Read the model definition and answer for the solid it produces. Units are mm, in the model's axes. A direction names the side the tool comes from. Give positions to 0.01 mm unless a question says otherwise; leave off trailing zeros. Order: outer loops, then holes, each group sorted by start corner. A loop starts at its lowest first (then second) coordinate and runs counter-clockwise, first axis right, second up. Notation, with made-up numbers: (17, -6.75) - (59, -6.75) arc R27 ccw to (59, 14.25) - close; hole circle Ø5 at (74, 31). An arc over 180 degrees is marked (long way). Write each question's results on one line, items separated by ' | '.
from build123d import *

# Parameters (mm, degrees)
F1_DEPTH = 127
F2_R     = 5.08
F4_DEPTH = 25.4
F5_R     = 3.9624
F6_DEPTH = 25.4


with BuildPart() as f1:
    # F0 (on Front) → F1 (new body, symmetric)
    with BuildSketch(Plane.XZ):
        Polygon((0, 152.4), (0, 0), (76.2, 0), (76.2, 9.525), (9.525, 9.525), (9.525, 152.4), align=None)
    extrude(amount=F1_DEPTH, both=True)

    # F2
    f2_edges = [f1.edges().sort_by_distance(p)[0] for p in [
        (9.525, 0, 152.4),
        (9.525, 0, 9.525),
        (76.2, 0, 9.525),
    ]]
    fillet(f2_edges, radius=F2_R)

    # F3 (on face) → F4 (cut)
    with BuildSketch(Plane(origin=(0, 0, 0), x_dir=(0, -1, 0), z_dir=(-1, 0, 0))):
        with BuildLine():
            Line((-90.4875, 104.775), (-90.4875, 120.65))
            ThreePointArc((-90.4875, 120.65), (-98.425, 128.5875), (-106.3625, 120.65))
            Line((-106.3625, 120.65), (-106.3625, 104.775))
            ThreePointArc((-106.3625, 104.775), (-98.425, 96.8375), (-90.4875, 104.775))
        make_face()
        with BuildLine():
            ThreePointArc((106.3625, 120.65), (98.425, 128.5875), (90.4875, 120.65))
            Line((90.4875, 120.65), (90.4875, 104.775))
            ThreePointArc((90.4875, 104.775), (98.425, 96.8375), (106.3625, 104.775))
            Line((106.3625, 104.775), (106.3625, 120.65))
        make_face()
    extrude(amount=-F4_DEPTH, mode=Mode.SUBTRACT)

    # F5 (on face) → F6 (cut)
    with BuildSketch(Plane(origin=(0, 0, 0), x_dir=(1, 0, 0), z_dir=(0, 0, -1))):
        with Locations((38.1, -101.6)):
            Circle(F5_R)
        with Locations((38.1, 101.6)):
            Circle(F5_R)
    extrude(amount=-F6_DEPTH, mode=Mode.SUBTRACT)


solid = f1.part
(1) Consider probe 1 along Y at (x, z) = (38, 5); probe 2 along X at (y, z) = (101.6, 3.5); probe 3 along X at (y, z) = (-101, 4). Determine where each line is inside the solid, lowest interval first. Write a range as [from, to].
Conclusion:
probe 1: [-127, -105.56], [-97.64, 97.64], [105.56, 127] | probe 2: [0, 34.14], [42.06, 76.2] | probe 3: [0, 34.18], [42.02, 76.2]
(2) Section A-A (z = 111.5) is taken. Give the vertices of the cut face in (x, y) (1 decimal).
Conclusion:
outline: (0, -127) - (9.5, -127) - (9.5, -106.4) - (0, -106.4) - close; (0, -90.5) - (9.5, -90.5) - (9.5, 90.5) - (0, 90.5) - close; (0, 106.4) - (9.5, 106.4) - (9.5, 127) - (0, 127) - close
(3) Each of these flat-tipped pins is pushed along its axis until it touches: pin 1 (7 mm diameter, centred on x = 38.1, y = 101.6, fed in from +Z); pin 2 (10.5 mm diameter, centred on x = 38.1, y = -101.6, fed in from +Z) (3 decimals); pin 3 (10 mm diameter, centred on x = 44, y = 87, fed in from -Z); pin 4 (3 mm diameter, centred on y = 22.5, z = 111, fed in from +X) (3 decimals). Where does it stop, or does it pass through?
Conclusion:
pin 1: through | pin 2: z = 9.525 | pin 3: z = 0 | pin 4: x = 9.525
(4) Section D-D (y = -63.5) is taken. Give the vertices of the cut face in (x, z) (3 decimals), plus the area to 3 significant figures.
Conclusion:
outline: (0, 0) - (76.2, 0) - (76.2, 4.445) arc R5.08 ccw to (71.12, 9.525) - (14.605, 9.525) arc R5.08 cw to (9.525, 14.605) - (9.525, 147.32) arc R5.08 ccw to (4.445, 152.4) - (0, 152.4) - close | area: 2,080 mm^2
(5) The mould has two halves that part along Y. Classify faces 1 (the face through (7, -127, 48)), 2 (the face through (5, -90.488, 113)), 3 (the face through (10.974, 1.778, 11.053)), 4 (the face through (4.696, 98.25, 128.586)): pulls with the +Y half, pulls with the -Y half, needs draft (parallel to the pull), parting line crosses it, or undercut.
Conclusion:
face 1: pulls with the -Y half | face 2: undercut | face 3: needs draft | face 4: undercut
(6) Section C-C (y = -101.6) is taken. Give the vertices of the cut face in (x, z) (3 decimals), plus the area to 3 significant figures.
Conclusion:
outline: (0, 0) - (34.138, 0) - (34.138, 9.525) - (14.605, 9.525) arc R5.08 cw to (9.525, 14.605) - (9.525, 97.5) - (0, 97.5) - close; (0, 127.925) - (9.525, 127.925) - (9.525, 147.32) arc R5.08 ccw to (4.445, 152.4) - (0, 152.4) - close; (42.062, 0) - (76.2, 0) - (76.2, 4.445) arc R5.08 ccw to (71.12, 9.525) - (42.062, 9.525) - close | area: 1,720 mm^2
(7) For faces 5 (the face through (9.525, -2, 80)), 6 (the face through (4.7, 98.6, 96.84)), 7 (the face through (38, -2, 0)), determine the directions among +Z, -Z, +X, -X, +Y, -Y from which every point of the face is accessible in a straight line to the end or side of a thin tool.
Conclusion:
face 5: +Z, +X, +Y, -Y | face 6: +X, -X | face 7: -Z, +X, -X, +Y, -Y
(8) Section B-B (x = 38.1) is taken. Give the vertices of the cut face in (y, z) (3 decimals), plus the area to 3 significant figures.
Conclusion:
outline: (-127, 0) - (-105.562, 0) - (-105.562, 9.525) - (-127, 9.525) - close; (-97.638, 0) - (97.638, 0) - (97.638, 9.525) - (-97.638, 9.525) - close; (105.562, 0) - (127, 0) - (127, 9.525) - (105.562, 9.525) - close | area: 2,270 mm^2
